Design review of the part built by this model. Coordinates are the model's own, in mm. Face numbers are marked on the shaded views. Round coordinates to 2 decimals unless told otherwise and drop trailing zeros. Write each loop counter-clockwise with the first axis right and the second up, starting at its lowest first coordinate (ties: lowest second). Pieces come first, ordered by that corner, then holes. Notation, with made-up numbers: M 62,68.25 L 105,68.25 A24 ccw 105,87.25 Z; hole C 73,69 d11. An arc over 180 degrees is marked long. One line per question, with ' | ' between items. Start each with the question number.
Item 1: Draft analysis for pull direction Y (two halves, no side actions). For the marked faces 1, 2 and 3, state which applies: released by +Y, released by -Y, zero draft, split by the parting line, or undercut.
Item 2: Insertion check: pin 1 Ø5 at (y, z) = (92, -1.5) entering from -X; pin 2 Ø3.5 at (y, z) = (-28.5, 29.5) entering from -X; pin 3 Ø1.5 at (x, y) = (-39, 5) entering from -Z. Each pin has a flat end and moves straight along its axis. Give the tip position at first contact, or say it passes through.
Item 3: For L1, parallel to X at y = -16, z = 23.5; L2, parallel to X at y = -11.5, z = -7.5; L3, parallel to Y at x = 208, z = 36.5, list the stretches that pass through material, from the lowest coordinate up.
Item 4: Add section A-A, the plane x = 107.5. State the section outline as (y, z) points.
Item 5: Add section B-B, the plane y = -95.5. State the section outline as (x, z) points.
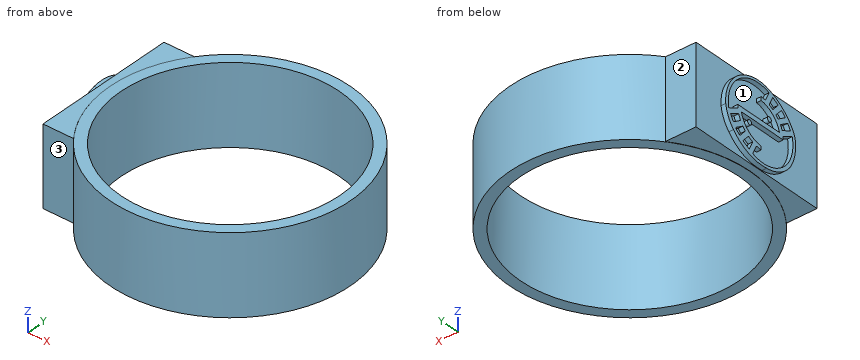
```python
from build123d import *

# Parameters (mm, degrees)
F0_W          = 11.7173120379
F0_H          = 86.0708840191
F3_DEPTH      = 62.484
F3_DEPTH_BACK = 23.114
F4_W          = 156.3523858786
F4_H          = 85.598
F4_R          = 2.5222307947
F5_DEPTH      = 5.08
F6_R          = 26.6100138709


# Not quite as in the source:
# - a feature names something its author has since deleted; it is built from what else it names


with BuildPart() as f1:
    # F0 (on Front) → F1 (revolve)
    with BuildSketch(Plane.XZ):
        with Locations((-22.7350816131, 19.6008179337)):
            Rectangle(F0_W, F0_H)
    revolve(axis=Axis((101.913869381, 0, 19.6008179337), (0, 0, -1)))

    # F2 (on Top) → F3 (join, two sides)
    with BuildSketch(Plane.XY) as f3_sk:
        Polygon((-23.8777473569, 0), (0, 78.1761929393), (-40.9507118165, 78.1761929393), (-40.9507118165, -78.1761929393), (0, -78.1761929393), align=None)
    extrude(amount=F3_DEPTH)
    extrude(f3_sk.sketch, amount=-F3_DEPTH_BACK)

    # F4 (on face) → F5 (cut)
    with BuildSketch(Plane(origin=(-40.9507118165, 0, 0), x_dir=(0, -1, 0), z_dir=(-1, 0, 0))):
        with Locations((0, 19.685)):
            Rectangle(F4_W, F4_H)
        with BuildLine():
            ThreePointArc((-45.8005852997, 15.4996816942), (-31.1457944751, 50.9769783822), (6.1403359286, 60.0954187045))
            ThreePointArc((6.1403359286, 60.0954187045), (28.1936749549, 48.849051517), (43.5657799244, 29.4446982443))
            ThreePointArc((43.5657799244, 29.4446982443), (43.8109995681, 11.2280239142), (37.0950251818, -5.7072364725))
            ThreePointArc((37.0950251818, -5.7072364725), (23.9203018158, -17.178744297), (7.161276415, -22.1086423844))
            ThreePointArc((7.161276415, -22.1086423844), (-16.4091184559, -19.3057274535), (-35.8321219683, -5.6614326371))
            ThreePointArc((-35.8321219683, -5.6614326371), (-42.4741077992, 4.1381986591), (-45.8005852997, 15.4996816942))
        make_face(mode=Mode.SUBTRACT)
        with BuildLine():
            Line((40.1134712131, 27.2007611227), (28.5185842412, 21.4439421826))
            Line((28.5185842412, 21.4439421826), (28.5185842412, 17.7521709857))
            Line((28.5185842412, 17.7521709857), (-25.6030233871, 17.7521709857))
            ThreePointArc((-25.6030233871, 17.7521709857), (-16.3053602602, 2.8665512096), (0, -3.6267871095))
            Line((0, -3.6267871095), (0, -7.4742618075))
            ThreePointArc((0, -7.4742618075), (-3.0208305793, -7.2095008507), (-6.0036519209, -6.6633391553))
            Line((-6.0036519209, -6.6633391553), (-10.9303286299, -16.9180645665))
            ThreePointArc((-10.9303286299, -16.9180645665), (27.850277377, -10.1984693401), (40.1134712131, 27.2007611227))
        make_face()
        with Locations((-14.9526894093, 12.6375420892)):
            Circle(F4_R, mode=Mode.SUBTRACT)
        with BuildLine():
            Line((-30.2748965285, 18.925355512), (-30.2748965285, 22.6689743163))
            Line((-30.2748965285, 22.6689743163), (23.6969497055, 22.6689743163))
            ThreePointArc((23.6969497055, 22.6689743163), (14.8585733056, 36.2512107395), (0, 42.7178051265))
            Line((0, 42.7178051265), (0, 46.5652798245))
            ThreePointArc((0, 46.5652798245), (2.7362509253, 46.2128562393), (5.4325754525, 45.6288138147))
            Line((5.4325754525, 45.6288138147), (10.3592521615, 55.8835392259))
            ThreePointArc((10.3592521615, 55.8835392259), (-28.2973985554, 49.8617154144), (-41.8697835003, 13.1685365719))
            Line((-41.8697835003, 13.1685365719), (-30.2748965285, 18.925355512))
        make_face()
        with Locations((10.5805564672, 29.0767555067)):
            Circle(F4_R, mode=Mode.SUBTRACT)
        with BuildLine():
            ThreePointArc((-23.5536272178, -10.4727910391), (-19.567339601, -12.673386574), (-15.5009556321, -14.7221986906))
            Line((-15.5009556321, -14.7221986906), (-10.8854688828, -5.1152055697))
            ThreePointArc((-10.8854688828, -5.1152055697), (-13.7327556617, -3.7930202048), (-16.4386400958, -2.2013526611))
            Line((-16.4386400958, -2.2013526611), (-23.5536272178, -10.4727910391))
        make_face()
        with BuildLine():
            ThreePointArc((-26.5336921008, 8.3536629544), (-27.9587005711, 11.0330778371), (-29.1266296715, 13.8341231545))
            Line((-29.1266296715, 13.8341231545), (-39.6148164121, 8.6267768283))
            ThreePointArc((-39.6148164121, 8.6267768283), (-37.8198393057, 5.3233394517), (-35.7862055506, 2.1612238524))
            Line((-35.7862055506, 2.1612238524), (-26.5336921008, 8.3536629544))
        make_face()
        with BuildLine():
            ThreePointArc((22.037269041, 49.3868926394), (18.5082065055, 51.5635703889), (14.8724930701, 53.5570086801))
            Line((14.8724930701, 53.5570086801), (10.2570063209, 43.9500155592))
            ThreePointArc((10.2570063209, 43.9500155592), (12.731329703, 42.7351985505), (15.0933792595, 41.3143613127))
            Line((15.0933792595, 41.3143613127), (22.037269041, 49.3868926394))
        make_face()
        with BuildLine():
            ThreePointArc((24.8030604194, 31.2912532728), (26.1088071334, 28.9630296891), (27.2183651143, 26.5351745401))
            Line((27.2183651143, 26.5351745401), (37.7065518548, 31.7425208664))
            ThreePointArc((37.7065518548, 31.7425208664), (36.0872429679, 34.7420367782), (34.1578114173, 37.5521170028))
            Line((34.1578114173, 37.5521170028), (24.8030604194, 31.2912532728))
        make_face()
        with BuildLine():
            ThreePointArc((-20.4539452974, 0.9064794757), (-22.0908205991, 2.5015221962), (-23.6111177136, 4.2080446007))
            Line((-23.6111177136, 4.2080446007), (-32.9658687115, -2.0528191293))
            ThreePointArc((-32.9658687115, -2.0528191293), (-30.4877258305, -4.9425156474), (-27.3978350789, -7.166051851))
            Line((-27.3978350789, -7.166051851), (-20.4539452974, 0.9064794757))
        make_face()
        with BuildLine():
            ThreePointArc((19.0953313845, 38.1919350162), (20.4937445485, 36.8328627443), (21.8078204864, 35.3920847438))
            Line((21.8078204864, 35.3920847438), (31.0603339362, 41.5845238458))
            ThreePointArc((31.0603339362, 41.5845238458), (28.7909533219, 44.1786559607), (26.2103185065, 46.4633733942))
            Line((26.2103185065, 46.4633733942), (19.0953313845, 38.1919350162))
        make_face()
    extrude(amount=-F5_DEPTH, mode=Mode.SUBTRACT)

    # F6
    f6_edges = [f1.edges().sort_by_distance(p)[0] for p in [
        (-38.410712, -43.56578, 29.444698),
    ]]
    fillet(f6_edges, radius=F6_R)


solid = f1.part
```
Computed values:
1) face 1: undercut | face 2: released by +Y | face 3: released by -Y
2) pin 1: stops at x = 6.93 | pin 2: stops at x = -35.87 | pin 3: stops at z = -22.23
3) L1: x = -35.87 to -15.79, 219.62 to 231.44 | L2: x = -35.87 to -16.32, 220.15 to 231.91 | L3: y = -76.01 to -53.45, 53.45 to 76.01
4) outline: M -130.39,-23.43 L -118.66,-23.43 L -118.66,62.64 L -130.39,62.64 Z; M 118.66,-23.43 L 130.39,-23.43 L 130.39,62.64 L 118.66,62.64 Z
5) outline: M 12.96,-23.43 L 31.27,-23.43 L 31.27,62.64 L 12.96,62.64 Z; M 172.56,-23.43 L 190.86,-23.43 L 190.86,62.64 L 172.56,62.64 Z
